Check sheet for the modelled part. Datum: model origin and axes. Units: mm. Face numbers are marked on the shaded views. A direction names the side the tool comes from. Coordinates: 2 decimals unless noted, no trailing zeros. Loops run counter-clockwise (first coordinate to the right, second up) from the corner with the lowest first, then second, coordinate; pieces in that order, holes last. Notation, with made-up numbers: (-6, -11.75) - (20, -11.75) arc R5 ccw to (20, -6.75) - close; hole circle Ø11 at (-26.5, -35.5). An arc over 180 degrees is marked (long way). Use a Markdown table: item, result. Add a question column.
1) Thickness scan on line 1 (X direction, y = 27.6, z = 43); line 2 (Z direction, x = 20, y = 26); line 3 (Y direction, x = -13.5, z = 21.5). Record the ranges inside material, lowest first.
2) Sectioned sample at A-A, the plane x = 20. Enter the section's corners in (y, z).
3) Sectioned sample at B-B, the plane z = 43. Enter the section's corners in (x, y), then the cut area to 3 significant figures.
4) Go/stop test with flat-tipped pins: P1, Ø10, axis at y = -1, z = 19.5, coming from the +X side; P2, Ø16.5, axis at x = -4, y = -1.5, coming from the -Z side; P3, Ø8, axis at x = -22.5, y = -6, coming from the -Z side; P4, Ø1.5, axis at y = 27.5, z = 38.5, coming from the +X side. Record where each tip stops, or that it passes through.
5) Sectioned sample at C-C, the plane z = 22.5. Enter the section's corners in (x, y).
6) Draft check along Y on the marked faces 1, 2 and 3. Enter one of: pulls with the +Y half, pulls with the -Y half, needs draft (parallel to the pull), parting line crosses it, or undercut.
7) Tool access check on the marked faces 4, 5 and 6. Record the directions out of +Z, -Z, +X, -X, +Y, -Y that give a thin tool (end or side, any length) a straight path to the whole face; none if there is none.
8) Sectioned sample at D-D, the plane y = 0.5. Enter the section's corners in (x, z), then the cut area to 3 significant figures.
from build123d import *

# Parameters (mm, degrees)
SKETCH_2_W          = 70
SKETCH_2_H          = 60
EXTRUDE_2_DEPTH     = 33
SKETCH_3_W          = 40.7
SKETCH_3_H          = 20.5
CUT_EXTRUDE_1_DEPTH = 28
SKETCH_4_W          = 14.65
SKETCH_4_H          = 20.5
EXTRUDE_3_DEPTH     = 28
SKETCH_5_W          = 14.65
SKETCH_5_H          = 20.5
CUT_EXTRUDE_4_DEPTH = 28
SKETCH_8_W          = 10
SKETCH_8_H          = 5
EXTRUDE_5_DEPTH     = 50
M3X0_5_1_D          = 2.5


with BuildPart() as part:
    # ｽｹｯﾁ2 → ﾎﾞｽ - 押し出し2 (new body)
    with BuildSketch(Plane.XY):
        Rectangle(SKETCH_2_W, SKETCH_2_H)
    extrude(amount=EXTRUDE_2_DEPTH)

    # ｽｹｯﾁ3 → ｶｯﾄ - 押し出し1 (cut)
    with BuildSketch(Plane.XY):
        Rectangle(SKETCH_3_W, SKETCH_3_H)
    extrude(amount=CUT_EXTRUDE_1_DEPTH, mode=Mode.SUBTRACT)

    # ｽｹｯﾁ4 → ﾎﾞｽ - 押し出し3 (add)
    with BuildSketch(Plane.XY):
        with Locations((27.675, 0)):
            Rectangle(SKETCH_4_W, SKETCH_4_H)
    extrude(amount=EXTRUDE_3_DEPTH)

    # ｽｹｯﾁ5 → ｶｯﾄ - 押し出し4 (cut)
    with BuildSketch(Plane.XY):
        with Locations((27.675, 0)):
            Rectangle(SKETCH_5_W, SKETCH_5_H)
    extrude(amount=CUT_EXTRUDE_4_DEPTH, mode=Mode.SUBTRACT)

    # ｽｹｯﾁ8 → ﾎﾞｽ - 押し出し5 (add)
    with BuildSketch(Plane.XY):
        with Locations((-20, 27.5)):
            Rectangle(SKETCH_8_W, SKETCH_8_H)
        with Locations((20, 27.5)):
            Rectangle(SKETCH_8_W, SKETCH_8_H)
    extrude(amount=EXTRUDE_5_DEPTH)

    # M3x0.5 ねじ穴1 (through all)
    with Locations(Plane(origin=(0, 30, 0), x_dir=(1, 0, 0), z_dir=(0, 1, 0))):
        with Locations((-20, -43), (20, -43)):
            Hole(M3X0_5_1_D / 2)


solid = part.part
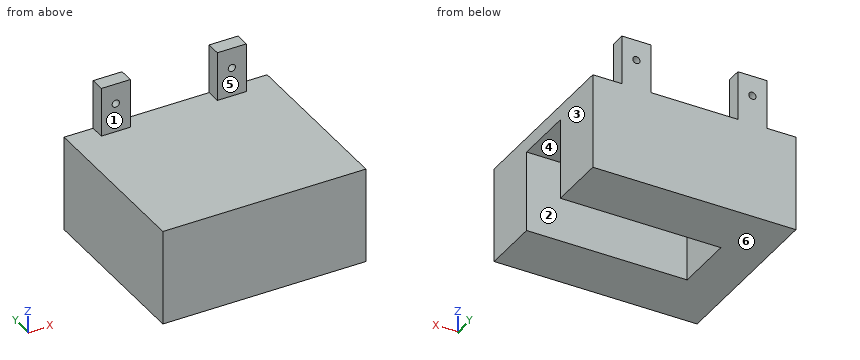
Solved:
| question | item | result |
|---|---|---|
| 1 | line 1 | x = -25 to -21.25, -18.75 to -15, 15 to 18.75, 21.25 to 25 |
| 1 | line 2 | z = 0 to 41.75, 44.25 to 50 |
| 1 | line 3 | y = -30 to -10.25, 10.25 to 30 |
| 2 | outline | (-30, 0) - (-10.25, 0) - (-10.25, 28) - (10.25, 28) - (10.25, 0) - (30, 0) - (30, 41.75) - (25, 41.75) - (25, 33) - (-30, 33) - close; (25, 44.25) - (30, 44.25) - (30, 50) - (25, 50) - close |
| 3 | outline | (-25, 25) - (-21.25, 25) - (-21.25, 30) - (-25, 30) - close; (-18.75, 25) - (-15, 25) - (-15, 30) - (-18.75, 30) - close; (15, 25) - (18.75, 25) - (18.75, 30) - (15, 30) - close; (21.25, 25) - (25, 25) - (25, 30) - (21.25, 30) - close |
| 3 | area | 75.0 mm2 |
| 4 | P1 | stops at x = -20.35 |
| 4 | P2 | stops at z = 28 |
| 4 | P3 | stops at z = 0 |
| 4 | P4 | stops at x = 25 |
| 5 | outline | (-35, -30) - (35, -30) - (35, -10.25) - (-20.35, -10.25) - (-20.35, 10.25) - (35, 10.25) - (35, 30) - (-35, 30) - close |
| 6 | face 1 | pulls with the -Y half |
| 6 | face 2 | undercut |
| 6 | face 3 | needs draft |
| 7 | face 4 | -Z, +X |
| 7 | face 5 | +Z, +X, -X, -Y |
| 7 | face 6 | -Z, +X, -X, +Y, -Y |
| 8 | outline | (-35, 0) - (-20.35, 0) - (-20.35, 28) - (35, 28) - (35, 33) - (-35, 33) - close |
| 8 | area | 760 mm2 |
